Work out the finished part from the listing and answer in its coordinate system (mm). Face numbers are marked on the shaded views. A direction names the side the tool comes from. Round coordinates to 2 decimals unless told otherwise and drop trailing zeros. Write each loop counter-clockwise with the first axis right and the second up, starting at its lowest first coordinate (ties: lowest second). Pieces come first, ordered by that corner, then holes.
1. Find section B-B (y = 14.5). Write down the section's boundary in (x, z).
2. A tool of negligible diameter and unlimited length cuts with its end or side. For the marked faces 1 and 2, from which of +Z, -Z, +X, -X, +Y, -Y can it reach the whole face along a straight path? Write none if from no direction.
3. Find section A-A (x = 4). Write down the section's boundary in (y, z).
4. Find section C-C (z = 18.5). Write down the section's boundary in (x, y), and give its area (3 significant figures).
5. Straight lines are drawn through the part: probe 1 along Z at (x, y) = (0.5, 13.75); probe 2 along Y at (x, z) = (8.25, 29.5); probe 3 along Y at (x, z) = (0.75, 14.5). For each, find the intervals that lie inside material, in ascending order.
6. Determine the mould class of the marked faces 3, 4, 5 and 6 for opening direction Y: pulls with the +Y half, pulls with the -Y half, needs draft (parallel to the pull), parting line crosses it, or undercut.
7. Flat-ended cylindrical pins translate along their axes: pin 1 Ø3 at (x, z) = (15, 27) entering from -Y; pin 2 Ø2 at (x, y) = (9.29, 9.1) entering from +Z; pin 3 Ø6 at (x, y) = (9, 13) entering from -Z; pin 4 Ø3 at (x, z) = (13, 25) entering from +Y. Find the tip coordinate at first contact, or state that the pin passes through.
```python
from build123d import *

# Parameters (mm, degrees)
BOSS_EXTRUDE1_DEPTH            = 33
SKETCH2_R                      = 2.75
BOSS_EXTRUDE2_DEPTH            = 3.1
M3_CLEARANCE_HOLE1_D           = 3.4
M3_CLEARANCE_HOLE1_DEPTH       = 3
M3_CLEARANCE_HOLE1_CSINK_D     = 3.45
M3_CLEARANCE_HOLE1_CSINK_ANGLE = 90
M3_CLEARANCE_HOLE1_TIP         = 1.021463052


with BuildPart() as part:
    # Sketch1 → Boss-Extrude1 (new body)
    with BuildSketch(Plane.XY):
        Polygon((17.123869681, -2.982979073), (21.366510368, 1.259661614), (1.447312342, 21.17885964), (-2.795328345, 16.936218953), align=None)
    extrude(amount=BOSS_EXTRUDE1_DEPTH)

    # Sketch2 → Boss-Extrude2 (add)
    with BuildSketch(Plane.XY.offset(33)):
        with Locations(Location((2.048353106, 16.335178189, 0), (0, 0, 180))):
            Circle(SKETCH2_R)
        with Locations(Location((16.522828917, 1.860702378, 0), (0, 0, 180))):
            Circle(SKETCH2_R)
    extrude(amount=BOSS_EXTRUDE2_DEPTH)

    # M3 Clearance Hole1
    with Locations(Plane.XY.offset(33)):
        with Locations((9.285591012, 9.097940284)):
            CounterSinkHole(M3_CLEARANCE_HOLE1_D / 2, M3_CLEARANCE_HOLE1_CSINK_D / 2, depth=M3_CLEARANCE_HOLE1_DEPTH, counter_sink_angle=M3_CLEARANCE_HOLE1_CSINK_ANGLE)
            with Locations((0, 0, -(M3_CLEARANCE_HOLE1_DEPTH + M3_CLEARANCE_HOLE1_TIP / 2))):  # 118° drill point
                Cone(0, M3_CLEARANCE_HOLE1_D / 2, M3_CLEARANCE_HOLE1_TIP, mode=Mode.SUBTRACT)


solid = part.part
```
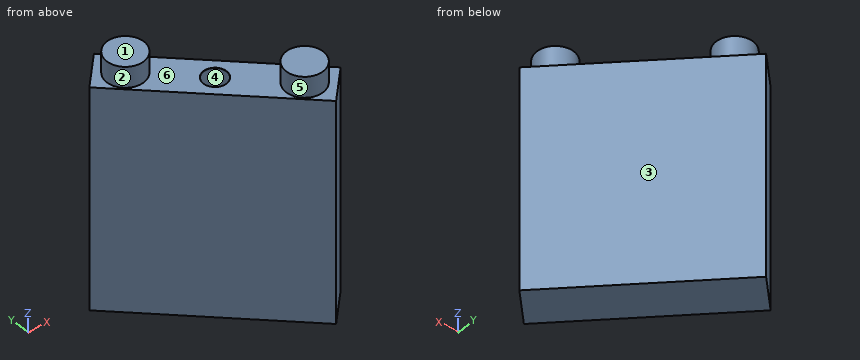
Worked answers:
1. outline: (-0.36, 0) - (8.13, 0) - (8.13, 33) - (4.1, 33) - (4.1, 36.1) - (0, 36.1) - (0, 33) - (-0.36, 33) - close
2. face 1: +Z, +X, -X, +Y, -Y
2. face 2: +Z
3. outline: (10.14, 0) - (18.63, 0) - (18.63, 33) - (18.27, 33) - (18.27, 36.1) - (14.4, 36.1) - (14.4, 33) - (10.14, 33) - close
4. outline: (-2.8, 16.94) - (17.12, -2.98) - (21.37, 1.26) - (1.45, 21.18) - close
4. area: 169 mm2
5. probe 1: z = 0 to 33
5. probe 2: y = 5.89 to 14.38
5. probe 3: y = 13.39 to 20.48
6. face 3: pulls with the +Y half
6. face 4: undercut
6. face 5: parting line crosses it
6. face 6: needs draft
7. pin 1: stops at y = -2.36
7. pin 2: stops at z = 29.58
7. pin 3: stops at z = 0
7. pin 4: stops at y = 11.13
